The figure shows three views and two pictorial views of one solid part (mm, origin at its lowest corner). Answer the questions. A direction names the side the tool comes from. Give positions to 0.01 mm unless a question says otherwise; leave off trailing zeros. Write each loop counter-clockwise with the first axis right and the second up, starting at its lowest first coordinate (ties: lowest second). Pieces come first, ordered by that corner, then holes. Notation, with made-up numbers: (34.5, 62) -> (81.5, 62) arc R38 ccw to (81.5, 101) -> close; hole circle Ø4 at (-27, -14.5). An arc over 180 degrees is marked (long way). Use a Markdown table: item, result.
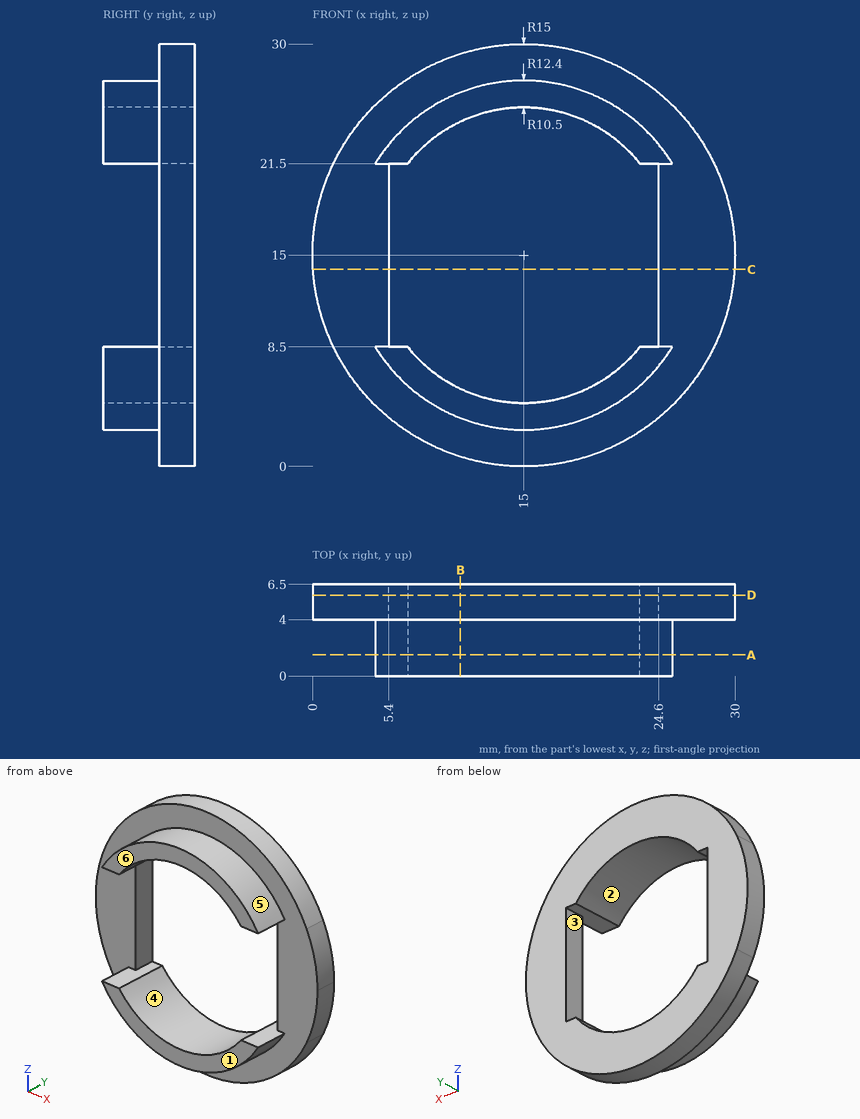
Item 1: A tool of negligible diameter and unlimited length cuts with its end or side. For the marked faces 1 and 2, from which of +Z, -Z, +X, -X, +Y, -Y can it reach the whole face along a straight path? Write none if from no direction.
Return value:
| item | result |
|---|---|
| face 1 | +Z, -Z, +X, -X, -Y |
| face 2 | +Y, -Y |
Item 2: Each of these flat-tipped pins is pushed along its axis until it touches: P1, Ø1.9, axis at x = 5.5, y = 2.5, coming from the -Z side; P2, Ø0.7, axis at x = 24, y = 4.5, coming from the -Z side; P3, Ø0.8, axis at y = 5.5, z = 16.5, coming from the -X side. Where does it stop, or does it pass through?
Return value:
| item | result |
|---|---|
| P1 | z = 6.02 |
| P2 | z = 2.75 |
| P3 | x = 0.04 |
Item 3: A cutting plane is placed at A-A (y = 1.5). Give the vertices of the cut face in (x, z).
Return value:
| item | result |
|---|---|
| outline | (4.44, 8.5) arc R12.4 ccw to (25.56, 8.5) -> (23.25, 8.5) arc R10.5 cw to (6.75, 8.5) -> close; (4.44, 21.5) -> (6.75, 21.5) arc R10.5 cw to (23.25, 21.5) -> (25.56, 21.5) arc R12.4 ccw to start |
Item 4: A cutting plane is placed at D-D (y = 5.75). Give the vertices of the cut face in (x, z).
Return value:
| item | result |
|---|---|
| outline | circle Ø30 at (15, 15); hole (5.4, 8.5) -> (6.75, 8.5) arc R10.5 ccw to (23.25, 8.5) -> (24.6, 8.5) -> (24.6, 21.5) -> (23.25, 21.5) arc R10.5 ccw to (6.75, 21.5) -> (5.4, 21.5) -> close |
Item 5: A cutting plane is placed at B-B (x = 10.5). Give the vertices of the cut face in (y, z), then the cut area to 3 significant figures.
Return value:
| item | result |
|---|---|
| outline | (0, 3.45) -> (4, 3.45) -> (4, 0.69) -> (6.5, 0.69) -> (6.5, 5.51) -> (0, 5.51) -> close; (0, 24.49) -> (6.5, 24.49) -> (6.5, 29.31) -> (4, 29.31) -> (4, 26.55) -> (0, 26.55) -> close |
| area | 40.7 mm^2 |
Item 6: For a pull along Z with two mould halves and no side action, classify the marked faces 3, 4, 5 and 6 as +Z half, -Z half, draft (parallel to the pull), parting line (faces both ways), or undercut.
Return value:
| item | result |
|---|---|
| face 3 | undercut |
| face 4 | undercut |
| face 5 | +Z half |
| face 6 | draft |
Item 7: Straight lines are drawn through the part: line 1 along Z through (x, y) = (5.5, 0.5); line 2 along Y through (x, z) = (25.5, 5); line 3 along X through (y, z) = (0.5, 22.25). For each, find the intervals that lie inside material, in ascending order. Write a range as [from, to].
Return value:
| item | result |
|---|---|
| line 1 | [7.03, 8.5], [21.5, 22.97] |
| line 2 | [4, 6.5] |
| line 3 | [4.94, 7.4], [22.6, 25.06] |
Item 8: A cutting plane is placed at C-C (z = 14). Give the vertices of the cut face in (x, y).
Return value:
| item | result |
|---|---|
| outline | (0.03, 4) -> (5.4, 4) -> (5.4, 6.5) -> (0.03, 6.5) -> close; (24.6, 4) -> (29.97, 4) -> (29.97, 6.5) -> (24.6, 6.5) -> close |
